Can you work these out from the drawing? Everything is in mm from the part's minimum corner. Coordinates: 2 decimals unless noted, no trailing zeros. Loops run counter-clockwise (first coordinate to the right, second up) from the corner with the lowest first, then second, coordinate; pieces in that order, holes last. Notation, with made-up numbers: M -37,-34 L 9,-34 A4 ccw 9,-29 Z; hole C -35,84 d10. An arc over 180 degrees is marked long. Use CSV: the item, a comma, the result in double quotes. Start each with the question number.
Q1. For pin 1 Ø3 at (x, z) = (77.27, 12.7) entering from +Y, with a flat end and sliding along its axis, tell me the tip position at first contact or that it passes through.
Q2. If we section it at A-A (x = 12.7): Please give me the cut outline in (y, z) (3 decimals).
Q3. If we mould it in two halves opening along Y, with no side actions, what happens to the marked faces 1 and 2? For each: +Y half, -Y half, draft (parallel to the pull), parting line (faces both ways), or undercut.
Q4. If we section it at B-B (y = 1.1): State how many separate pieces and enclosed holes the cut face has, and give its area (3 significant figures).
Q5. If we section it at C-C (z = 12.7): Please give me the cut outline in (x, y) (1 decimal).
Q6. Please list where these lines run through material, in increasing order: probe 1 along X at (y, z) = (1.2, 12.7) (1 decimal); probe 2 along Z at (x, y) = (12.7, 1.1) (3 decimals); probe 3 along X at (y, z) = (0.8, 11). Write a range as [from, to].
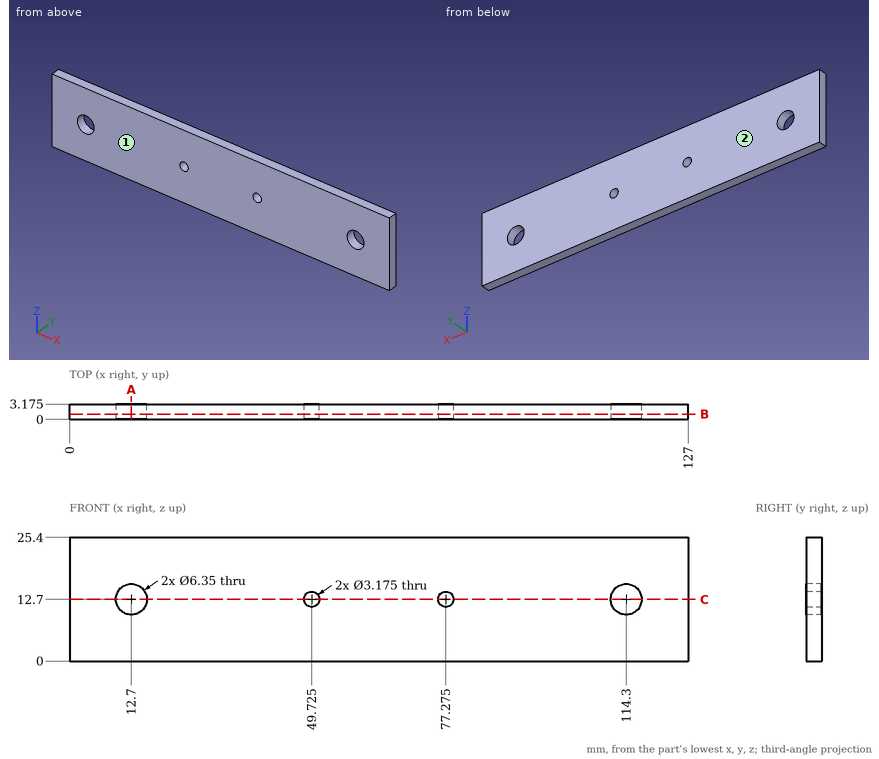
Results below:
1,pin 1,"through"
2,outline,"M 0,0 L 3.175,0 L 3.175,9.525 L 0,9.525 Z; M 0,15.875 L 3.175,15.875 L 3.175,25.4 L 0,25.4 Z"
3,face 1,"-Y half"
3,face 2,"+Y half"
4,separate pieces,"1"
4,enclosed holes,"4"
4,area,"3,150 mm^2"
5,outline,"M 0,0 L 9.5,0 L 9.5,3.2 L 0,3.2 Z; M 15.9,0 L 48.1,0 L 48.1,3.2 L 15.9,3.2 Z; M 51.3,0 L 75.7,0 L 75.7,3.2 L 51.3,3.2 Z; M 78.9,0 L 111.1,0 L 111.1,3.2 L 78.9,3.2 Z; M 117.5,0 L 127,0 L 127,3.2 L 117.5,3.2 Z"
6,probe 1,"[0, 9.5], [15.9, 48.1], [51.3, 75.7], [78.9, 111.1], [117.5, 127]"
6,probe 2,"[0, 9.525], [15.875, 25.4]"
6,probe 3,"[0, 10.02], [15.38, 111.62], [116.98, 127]"
